Geometry: final body of the model. Coordinates: model frame, mm. Face numbers are marked on the shaded views. Give positions to 0.01 mm unless a question says otherwise; leave off trailing zeros. Write each loop counter-clockwise with the first axis right and the second up, starting at its lowest first coordinate (ties: lowest second). Pieces come first, ordered by that corner, then holes. Notation, with made-up numbers: (0.25, -13) - (48.25, -13) arc R26 ccw to (48.25, 15) - close; hole circle Ø1 at (52.5, 81). An arc over 180 degrees is marked (long way). Use CSV: the item, a comma, the result in double quotes. Start each with the question number.
(1) Line query: probe 1 along Z at (x, y) = (213, -402); probe 2 along Y at (x, z) = (153, 82); probe 3 along X at (y, z) = (-289, 70). Output: solid intervals per line, ascending. Write a range as [from, to].
(2) Section D-D on z = 180.5. Output: boundary loops of the cut face in (x, y).
(3) Draft query along X for the marked faces 1, 2 and 3. Return one class per face: released by +X, released by -X, zero draft, split by the parting line, or undercut.
(4) Section B-B on z = 33.5. Output: boundary loops of the cut face in (x, y).
(5) First-contact query: pin 1 Ø4 at (x, y) = (35.5, -164) entering from +Z; pin 2 Ø2 at (y, z) = (-539, 170.5) entering from +X; pin 3 Ø1.2 at (y, z) = (-537.5, 164.5) entering from -X. Flat tips, straight axial feed; report the tip coordinate or a pass-through.
(6) Section C-C on x = 91.5. Output: boundary loops of the cut face in (y, z).
(7) Section A-A on y = -235.5. Output: boundary loops of the cut face in (x, z), and give its area (3 significant figures).
from build123d import *

# Parameters (mm, degrees)
ESQUISSE1_W             = 235
ESQUISSE1_H             = 540
BOSS_EXTRU_1_DEPTH      = 145
ESQUISSE2_W             = 227
ESQUISSE2_H             = 532
ENL_V_MAT_EXTRU_1_DEPTH = 141
ESQUISSE3_W             = 235
ESQUISSE3_H             = 540
BOSS_EXTRU_2_DEPTH      = 4
ESQUISSE4_W             = 120
ESQUISSE4_H             = 70
ENL_V_MAT_EXTRU_2_DEPTH = 4
ESQUISSE5_W             = 120
ESQUISSE5_H             = 4
BOSS_EXTRU_3_DEPTH      = 70


with BuildPart() as part:
    # Esquisse1 → Boss.-Extru.1 (new body)
    with BuildSketch(Plane.XY):
        with Locations((117.5, -270)):
            Rectangle(ESQUISSE1_W, ESQUISSE1_H)
    extrude(amount=BOSS_EXTRU_1_DEPTH)

    # Esquisse2 → Enlèv. mat.-Extru.1 (cut)
    with BuildSketch(Plane.XY.offset(145)):
        with Locations((117.5, -270)):
            Rectangle(ESQUISSE2_W, ESQUISSE2_H)
    extrude(amount=-ENL_V_MAT_EXTRU_1_DEPTH, mode=Mode.SUBTRACT)

    # Esquisse3 → Boss.-Extru.2 (add)
    with BuildSketch(Plane.XY.offset(145)):
        with Locations((117.5, -270)):
            Rectangle(ESQUISSE3_W, ESQUISSE3_H)
    extrude(amount=-BOSS_EXTRU_2_DEPTH)

    # Esquisse4 → Enlèv. mat.-Extru.2 (cut)
    with BuildSketch(Plane.XY.offset(145)):
        with Locations((117.5, -501)):
            Rectangle(ESQUISSE4_W, ESQUISSE4_H)
    extrude(amount=-ENL_V_MAT_EXTRU_2_DEPTH, mode=Mode.SUBTRACT)

    # Esquisse5 → Boss.-Extru.3 (add)
    with BuildSketch(Plane.XY.offset(145)):
        with Locations((117.5, -538)):
            Rectangle(ESQUISSE5_W, ESQUISSE5_H)
    extrude(amount=BOSS_EXTRU_3_DEPTH)


solid = part.part
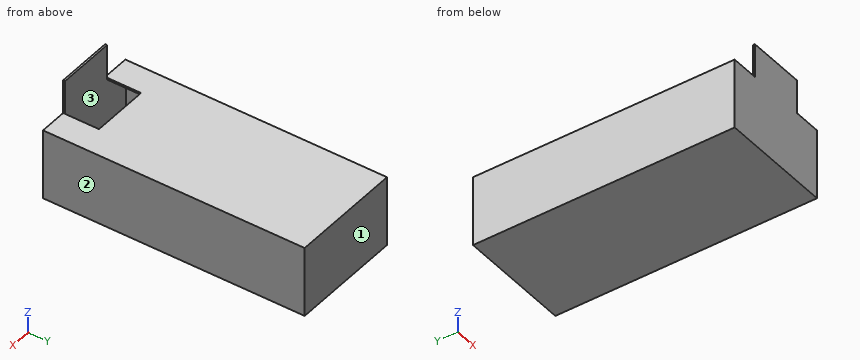
Check values:
1,probe 1,"z = [0, 4], [141, 145]"
1,probe 2,"y = [-540, -536], [-4, 0]"
1,probe 3,"x = [0, 4], [231, 235]"
2,outline,"(57.5, -540) - (177.5, -540) - (177.5, -536) - (57.5, -536) - close"
3,face 1,"zero draft"
3,face 2,"released by +X"
3,face 3,"undercut"
4,outline,"(0, -540) - (235, -540) - (235, 0) - (0, 0) - close; hole (4, -536) - (231, -536) - (231, -4) - (4, -4) - close"
5,pin 1,"stops at z = 145"
5,pin 2,"stops at x = 177.5"
5,pin 3,"stops at x = 57.5"
6,outline,"(-540, 0) - (0, 0) - (0, 145) - (-466, 145) - (-466, 141) - (-4, 141) - (-4, 4) - (-536, 4) - (-536, 215) - (-540, 215) - close"
7,outline,"(0, 0) - (235, 0) - (235, 145) - (0, 145) - close; hole (4, 4) - (231, 4) - (231, 141) - (4, 141) - close"
7,area,"2,980 mm²"
